Autodesk Inventor part; units mm, degrees
ref_plane "YZ Plane" through (0, 0, 0) normal (1, 0, 0) x (0, 1, 0)
ref_plane "XZ Plane" through (0, 0, 0) normal (0, 1, 0) x (-1, 0, 0)
ref_plane "XY Plane" through (0, 0, 0) normal (0, 0, 1) x (1, 0, 0)
sketch "Sketch1" plane through (0, 0, 0) normal (0, 0, 1) x (1, 0, 0)
  circle A0 centre (0, 0) radius 2.5
  circle A1 centre (0, 0) radius 1.5
  dimension "d0" = 5
  dimension "d1" = 3
extrude "Extrusion1" add sketch "Sketch1" along normal mid plane 30
thread "Thread1"
thread "Thread2"
chamfer "Chamfer1" distance 0.1 angle 45 4 edges at (-2.5, 0, 15) (-1.5, 0, 15) (-1.5, 0, -15) (-2.5, 0, -15)
properties part number "M3 30mm Standoff" material "Aluminum 6061"
Part model, mm, in its own coordinate system. Round coordinates to 2 decimals unless told otherwise and drop trailing zeros. Write each loop counter-clockwise with the first axis right and the second up, starting at its lowest first coordinate (ties: lowest second). Pieces come first, ordered by that corner, then holes. Notation, with made-up numbers: M -20,-12 L -12,-12 A15 cw -12,-7 Z; hole C 38,40.25 d2. An arc over 180 degrees is marked long. One line per question, with ' | ' between items.
(1) Saw through at C-C on z = 4.5. Write the cut outline in (x, y), then the cut area to 3 significant figures.
Answer key:
outline: C 0,0 d5; hole C 0,0 d3 | area: 12.6 mm^2
(2) Saw through at A-A on y = 0. Write the cut outline in (x, z).
Answer key:
outline: M -2.5,-14.9 L -2.4,-15 L -1.6,-15 L -1.5,-14.9 L -1.5,14.9 L -1.6,15 L -2.4,15 L -2.5,14.9 Z; M 1.5,-14.9 L 1.6,-15 L 2.4,-15 L 2.5,-14.9 L 2.5,14.9 L 2.4,15 L 1.6,15 L 1.5,14.9 Z
(3) Two-plate mould, pull along Y, no slides. Class faces 1 (the face through (0, -2, 15)), 2 (the face through (-1.5, 0.07, 0.21)), 3 (the face through (-0.54, 2.44, -0.21)): released by +Y, released by -Y, zero draft, split by the parting line, or undercut.
Answer key:
face 1: zero draft | face 2: undercut | face 3: split by the parting line
(4) Pin check, flat tips, straight feed: pin 1 (2.5 mm diameter, centred on x = 0, y = 0, fed in from -Z); pin 2 (1 mm diameter, centred on y = 1.5, z = 1, fed in from -X); pin 3 (1.5 mm diameter, centred on y = -2, z = -2, fed in from +X). Stop position of each tip, or through.
Answer key:
pin 1: passes through | pin 2: stops at x = -2.29 | pin 3: stops at x = 2.17
(5) Probe line 1 along Y through (x, z) = (0, 0.75); line 2 along X through (y, z) = (-1.15, -12.5); line 3 along X through (y, z) = (-1.35, 9.5). List the from-to ranges inside material, lowest first.
Answer key:
line 1: y = -2.5 to -1.5, 1.5 to 2.5 | line 2: x = -2.22 to -0.96, 0.96 to 2.22 | line 3: x = -2.1 to -0.65, 0.65 to 2.1
